```python
from build123d import *

# Parameters (mm, degrees)
F1_W     = 154.6539068222
F1_H     = 60.2537170053
F2_DEPTH = 25.4


with BuildPart() as f2:
    # F1 (on face) → F2 (new body)
    with BuildSketch(Plane.XY):
        with Locations((-1.9112378359, 44.7821803391)):
            Rectangle(F1_W, F1_H)
        with BuildLine():
            Line((-43.9133035187, 28.4521430731), (-47.2029023286, 28.4521430731))
            Line((-47.2029023286, 28.4521430731), (-48.0829768154, 32.6218163698))
            Line((-48.0829768154, 32.6218163698), (-48.2965871278, 32.6218163698))
            add(Edge.make_bspline(
                [(-48.2965871278, 32.6218163698), (-50.4839567261, 29.870515547), (-52.6585097056, 28.8921803165)],
                knots=[0, 0, 0, 1, 1, 1], degree=2))
            add(Edge.make_bspline(
                [(-52.6585097056, 28.8921803165), (-54.8330626851, 27.913845086), (-58.0970282576, 27.913845086)],
                knots=[0, 0, 0, 1, 1, 1], degree=2))
            add(Edge.make_bspline(
                [(-58.0970282576, 27.913845086), (-62.4461342167, 27.913845086), (-64.9154694272, 30.1610255717)],
                knots=[0, 0, 0, 1, 1, 1], degree=2))
            add(Edge.make_bspline(
                [(-64.9154694272, 30.1610255717), (-67.3848046378, 32.4082060575), (-67.3848046378, 36.5437017042)],
                knots=[0, 0, 0, 1, 1, 1], degree=2))
            add(Edge.make_bspline(
                [(-67.3848046378, 36.5437017042), (-67.3848046378, 45.4042574598), (-53.2096243114, 45.8314780844)],
                knots=[0, 0, 0, 1, 1, 1], degree=2))
            Line((-53.2096243114, 45.8314780844), (-48.2453206528, 45.9938219218))
            Line((-48.2453206528, 45.9938219218), (-48.2453206528, 47.8137817829))
            add(Edge.make_bspline(
                [(-48.2453206528, 47.8137817829), (-48.2453206528, 51.2571800177), (-49.7235040142, 52.8977072164)],
                knots=[0, 0, 0, 1, 1, 1], degree=2))
            add(Edge.make_bspline(
                [(-49.7235040142, 52.8977072164), (-51.2016873755, 54.5382344151), (-54.4656529479, 54.5382344151)],
                knots=[0, 0, 0, 1, 1, 1], degree=2))
            add(Edge.make_bspline(
                [(-54.4656529479, 54.5382344151), (-58.1226614951, 54.5382344151), (-62.7366442414, 52.2995983419)],
                knots=[0, 0, 0, 1, 1, 1], degree=2))
            Line((-62.7366442414, 52.2995983419), (-64.1037502404, 55.6917301017))
            add(Edge.make_bspline(
                [(-64.1037502404, 55.6917301017), (-61.9420138796, 56.8623146133), (-59.3658735128, 57.5287787878)],
                knots=[0, 0, 0, 1, 1, 1], degree=2))
            add(Edge.make_bspline(
                [(-59.3658735128, 57.5287787878), (-56.7897331461, 58.1952429622), (-54.1922317481, 58.1952429622)],
                knots=[0, 0, 0, 1, 1, 1], degree=2))
            add(Edge.make_bspline(
                [(-54.1922317481, 58.1952429622), (-48.9630513023, 58.1952429622), (-46.4381774105, 55.8754349703)],
                knots=[0, 0, 0, 1, 1, 1], degree=2))
            add(Edge.make_bspline(
                [(-46.4381774105, 55.8754349703), (-43.9133035187, 53.5556269784), (-43.9133035187, 48.4289794824)],
                knots=[0, 0, 0, 1, 1, 1], degree=2))
            Line((-43.9133035187, 48.4289794824), (-43.9133035187, 28.4521430731))
        make_face(mode=Mode.SUBTRACT)
        with BuildLine():
            add(Edge.make_bspline(
                [(17.8115323328, 29.4432949223), (14.8807988476, 27.913845086), (10.4206155261, 27.913845086)],
                knots=[0, 0, 0, 1, 1, 1], degree=2))
            add(Edge.make_bspline(
                [(10.4206155261, 27.913845086), (4.0635726311, 27.913845086), (0.5774523339, 31.8271860079)],
                knots=[0, 0, 0, 1, 1, 1], degree=2))
            add(Edge.make_bspline(
                [(0.5774523339, 31.8271860079), (-2.9086679634, 35.7405269299), (-2.9086679634, 42.9007445992)],
                knots=[0, 0, 0, 1, 1, 1], degree=2))
            add(Edge.make_bspline(
                [(-2.9086679634, 42.9007445992), (-2.9086679634, 50.240394931), (0.6329910151, 54.2477243903)],
                knots=[0, 0, 0, 1, 1, 1], degree=2))
            add(Edge.make_bspline(
                [(0.6329910151, 54.2477243903), (4.1746499935, 58.2550538497), (10.7111255509, 58.2550538497)],
                knots=[0, 0, 0, 1, 1, 1], degree=2))
            add(Edge.make_bspline(
                [(10.7111255509, 58.2550538497), (12.8215954367, 58.2550538497), (14.9320653226, 57.7979277813)],
                knots=[0, 0, 0, 1, 1, 1], degree=2))
            add(Edge.make_bspline(
                [(14.9320653226, 57.7979277813), (17.0425352084, 57.3408017129), (18.2387529575, 56.7256040134)],
                knots=[0, 0, 0, 1, 1, 1], degree=2))
            Line((18.2387529575, 56.7256040134), (16.8801913711, 52.9660625163))
            add(Edge.make_bspline(
                [(16.8801913711, 52.9660625163), (15.4105524222, 53.5556269784), (13.6760366861, 53.9401255406)],
                knots=[0, 0, 0, 1, 1, 1], degree=2))
            add(Edge.make_bspline(
                [(13.6760366861, 53.9401255406), (11.9415209499, 54.3246241028), (10.608592601, 54.3246241028)],
                knots=[0, 0, 0, 1, 1, 1], degree=2))
            add(Edge.make_bspline(
                [(10.608592601, 54.3246241028), (1.688225958, 54.3246241028), (1.688225958, 42.9520110742)],
                knots=[0, 0, 0, 1, 1, 1], degree=2))
            add(Edge.make_bspline(
                [(1.688225958, 42.9520110742), (1.688225958, 37.5604867909), (3.8627789375, 34.6767475744)],
                knots=[0, 0, 0, 1, 1, 1], degree=2))
            add(Edge.make_bspline(
                [(3.8627789375, 34.6767475744), (6.0373319171, 31.793008358), (10.3095381637, 31.793008358)],
                knots=[0, 0, 0, 1, 1, 1], degree=2))
            add(Edge.make_bspline(
                [(10.3095381637, 31.793008358), (13.9665467108, 31.793008358), (17.8115323328, 33.3651802567)],
                knots=[0, 0, 0, 1, 1, 1], degree=2))
            Line((17.8115323328, 33.3651802567), (17.8115323328, 29.4432949223))
        make_face(mode=Mode.SUBTRACT)
        with BuildLine():
            add(Edge.make_bspline(
                [(-30.3533208919, 53.8205037657), (-27.2602435693, 58.1952429622), (-21.1680774616, 58.1952429622)],
                knots=[0, 0, 0, 1, 1, 1], degree=2))
            add(Edge.make_bspline(
                [(-21.1680774616, 58.1952429622), (-15.4005990286, 58.1952429622), (-12.2092609624, 54.2562688028)],
                knots=[0, 0, 0, 1, 1, 1], degree=2))
            add(Edge.make_bspline(
                [(-12.2092609624, 54.2562688028), (-9.0179228961, 50.3172946434), (-9.0179228961, 43.1143549116)],
                knots=[0, 0, 0, 1, 1, 1], degree=2))
            add(Edge.make_bspline(
                [(-9.0179228961, 43.1143549116), (-9.0179228961, 35.9028707672), (-12.2348941998, 31.9083579266)],
                knots=[0, 0, 0, 1, 1, 1], degree=2))
            add(Edge.make_bspline(
                [(-12.2348941998, 31.9083579266), (-15.4518655036, 27.913845086), (-21.1680774616, 27.913845086)],
                knots=[0, 0, 0, 1, 1, 1], degree=2))
            add(Edge.make_bspline(
                [(-21.1680774616, 27.913845086), (-24.0304556468, 27.913845086), (-26.3929857012, 28.9690800289)],
                knots=[0, 0, 0, 1, 1, 1], degree=2))
            add(Edge.make_bspline(
                [(-26.3929857012, 28.9690800289), (-28.7555157556, 30.0243149718), (-30.3533208919, 32.2202289826)],
                knots=[0, 0, 0, 1, 1, 1], degree=2))
            Line((-30.3533208919, 32.2202289826), (-30.6780085666, 32.2202289826))
            Line((-30.6780085666, 32.2202289826), (-31.6093495284, 28.4521430731))
            Line((-31.6093495284, 28.4521430731), (-34.7878709759, 28.4521430731))
            Line((-34.7878709759, 28.4521430731), (-34.7878709759, 70.003621028))
            Line((-34.7878709759, 70.003621028), (-30.3533208919, 70.003621028))
            Line((-30.3533208919, 70.003621028), (-30.3533208919, 59.9041254609))
            add(Edge.make_bspline(
                [(-30.3533208919, 59.9041254609), (-30.3533208919, 56.5119937011), (-30.5669312042, 53.8205037657)],
                knots=[0, 0, 0, 1, 1, 1], degree=2))
            Line((-30.5669312042, 53.8205037657), (-30.3533208919, 53.8205037657))
        make_face(mode=Mode.SUBTRACT)
    extrude(amount=F2_DEPTH)


solid = f2.part
```
Model file for the job. Use its own axes, mm. A direction names the side the tool comes from. Coordinates: 2 decimals unless noted, no trailing zeros. Loops run counter-clockwise (first coordinate to the right, second up) from the corner with the lowest first, then second, coordinate; pieces in that order, holes last. Notation, with made-up numbers: (82.25, -18) - (133.25, -18) arc R20 cw to (133.25, 21) - close; hole circle Ø4 at (74, 42.5). An arc over 180 degrees is marked (long way). Answer as a JSON object with one key per item and string values. Group by question number.
(1) Tool access for faces 1 (the face through (-33, 28.452, 13)), 2 (the face through (-79.238, 44, 13)): list every direction of +Z, -Z, +X, -X, +Y, -Y with a clear straight run to the whole face (end or side of a thin tool).
(2) Probe line 1 along X through (y, z) = (61.5, 22.75); line 2 along Y through (x, z) = (-64, 7.75); line 3 along X through (y, z) = (40, 19). List the from-to ranges inside material, lowest first.
(3) Cut at A-A (y = 64). Give the cut face in (x, z).
(4) Cut at B-B (z = 23.75). State how many separate pieces and enclosed holes the cut face has, then the cut area to 3 significant figures.
(5) Two-plate mould, pull along X, no slides. Class faces 3 (the face through (75.416, 44, 13)), 4 (the face through (-3, 45, 25.4)), 5 (the face through (-34.788, 49, 13)): released by +X, released by -X, zero draft, split by the parting line, or undercut.
Geometry says:
{
 "1": {"face 1": "+Z, -Z", "face 2": "+Z, -Z, -X, +Y, -Y"},
 "2": {"line 1": "x = -79.24 to -34.79, -30.35 to 75.42", "line 2": "y = 14.66 to 29.45, 43.19 to 55.43, 55.75 to 74.91", "line 3": "x = -79.24 to -66.71, -43.91 to -34.79, -9.18 to -2.75, 1.88 to 75.42"},
 "3": {"outline": "(-79.24, 0) - (-34.79, 0) - (-34.79, 25.4) - (-79.24, 25.4) - close; (-30.35, 0) - (75.42, 0) - (75.42, 25.4) - (-30.35, 25.4) - close"},
 "4": {"separate pieces": "1", "enclosed holes": "3", "area": "7,890 mm^2"},
 "5": {"face 3": "released by +X", "face 4": "zero draft", "face 5": "undercut"}
}
